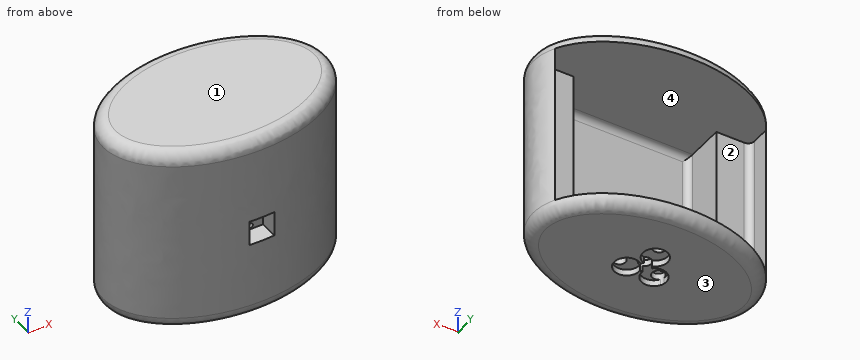
```python
from build123d import *

# Parameters (mm, degrees)
SKETCH1_RX               = 22.86
SKETCH1_RY               = 15.24
BOSS_EXTRUDE4_DEPTH      = 45.72
CUT_EXTRUDE2_START       = -10.16
SKETCH4_W                = 29.21
SKETCH4_H                = 17.78
CUT_EXTRUDE2_DEPTH       = 33.02
SKETCH7_W                = 14.643913221
SKETCH7_H                = 35.56
CUT_EXTRUDE4_DEPTH       = 33.02
CUT_EXTRUDE4_DEPTH_BACK  = 33.02
SKETCH8_R                = 1.27
CUT_EXTRUDE5_DEPTH       = 2.54
FILLET1_R                = 2.54
FILLET2_R                = 2.54
CUT_EXTRUDE11_START      = -2.54
SKETCH12_W               = 43.18
SKETCH12_H               = 19.05
CUT_EXTRUDE11_DEPTH      = 33.02
FILLET3_R                = 1.27
CUT_EXTRUDE13_START      = -2.54
SKETCH13_W               = 5.08
SKETCH13_H               = 5.08
CUT_EXTRUDE13_DEPTH      = 4.8100001
SKETCH14_R               = 0.5
CUT_EXTRUDE14_DEPTH      = 4.8100001
CUT_EXTRUDE14_DEPTH_BACK = 27.6700001
SKETCH16_R               = 2.54
CUT_EXTRUDE15_DEPTH      = 1.27
FILLET4_R                = 1.27


with BuildPart() as part:
    # Sketch1 → Boss-Extrude4 (new body)
    with BuildSketch(Plane.XY):
        with Locations(Location((0, 0), (0, 0, 180))):
            Ellipse(SKETCH1_RX, SKETCH1_RY)
    extrude(amount=BOSS_EXTRUDE4_DEPTH)

    # Sketch4 → Cut-Extrude2 (cut)
    with BuildSketch(Plane.XY.offset(45.72).offset(CUT_EXTRUDE2_START)):
        Rectangle(SKETCH4_W, SKETCH4_H)
    extrude(amount=-CUT_EXTRUDE2_DEPTH, mode=Mode.SUBTRACT)

    # Sketch7 → Cut-Extrude4 (cut, two sides)
    with BuildSketch(Plane(origin=(0, 0, 0), x_dir=(0, 0, -1), z_dir=(1, 0, 0))) as cut_extrude4_sk:
        with Locations((-45.421956611, -1.677648267)):
            Rectangle(SKETCH7_W, SKETCH7_H)
    extrude(amount=CUT_EXTRUDE4_DEPTH, mode=Mode.SUBTRACT)
    extrude(cut_extrude4_sk.sketch, amount=-CUT_EXTRUDE4_DEPTH_BACK, mode=Mode.SUBTRACT)

    # Sketch8 → Cut-Extrude5 (cut)
    with BuildSketch(Plane.XY):
        Circle(SKETCH8_R)
        with Locations((3.998447315, -1.999223657)):
            Circle(SKETCH8_R)
        with Locations((-3.998447315, -1.999223657)):
            Circle(SKETCH8_R)
        with Locations((0, 4.572)):
            Circle(SKETCH8_R)
    extrude(amount=CUT_EXTRUDE5_DEPTH, mode=Mode.SUBTRACT)

    # Fillet1
    fillet1_edges = [part.edges().sort_by_distance(p)[0] for p in [
        (22.859987041, 0.016227247, 0),
    ]]
    fillet(fillet1_edges, radius=FILLET1_R)

    # Fillet2
    fillet2_edges = [part.edges().sort_by_distance(p)[0] for p in [
        (22.860000074, 1.7e-08, 38.1),
    ]]
    fillet(fillet2_edges, radius=FILLET2_R)

    # Sketch12 → Cut-Extrude11 (cut)
    with BuildSketch(Plane(origin=(0, 0, 0), x_dir=(-1, 0, 0), z_dir=(0, 0, -1)).offset(CUT_EXTRUDE11_START)):
        with Locations((0, 9.525)):
            Rectangle(SKETCH12_W, SKETCH12_H)
    extrude(amount=-CUT_EXTRUDE11_DEPTH, mode=Mode.SUBTRACT)

    # Fillet3
    fillet3_edges = [part.edges().sort_by_distance(p)[0] for p in [
        (14.605, -8.89, 19.05),
        (0, -8.89, 35.56),
        (-14.605, -8.89, 19.05),
        (0, -8.89, 2.54),
    ]]
    fillet(fillet3_edges, radius=FILLET3_R)

    # Sketch13 → Cut-Extrude13 (cut, through all)
    with BuildSketch(Plane(origin=(0, -8.89, 0), x_dir=(1, 0, 0), z_dir=(0, 1, 0)).offset(CUT_EXTRUDE13_START)):
        with Locations((0, -18.288)):
            Rectangle(SKETCH13_W, SKETCH13_H)
    extrude(amount=-CUT_EXTRUDE13_DEPTH, mode=Mode.SUBTRACT)

    # Sketch14 → Cut-Extrude14 (cut, two sides)
    with BuildSketch(Plane.XZ.offset(11.43)) as cut_extrude14_sk:
        with Locations((0, 20.077999976)):
            Circle(SKETCH14_R)
        with Locations((0, 16.498)):
            Circle(SKETCH14_R)
    extrude(amount=CUT_EXTRUDE14_DEPTH, mode=Mode.SUBTRACT)
    extrude(cut_extrude14_sk.sketch, amount=-CUT_EXTRUDE14_DEPTH_BACK, mode=Mode.SUBTRACT)

    # Sketch16 → Cut-Extrude15 (cut)
    with BuildSketch(Plane(origin=(0, 0, 0), x_dir=(-1, 0, 0), z_dir=(0, 0, -1))):
        with Locations((2.7942426, -1.505997915)):
            Circle(SKETCH16_R)
        with Locations((0.000242604, 3.333352043)):
            Circle(SKETCH16_R)
        with Locations((-2.793757393, -1.505997915)):
            Circle(SKETCH16_R)
    extrude(amount=-CUT_EXTRUDE15_DEPTH, mode=Mode.SUBTRACT)

    # Fillet4
    fillet4_edges = [part.edges().sort_by_distance(p)[0] for p in [
        (-21.59, 0, 19.05),
        (21.59, 0, 19.05),
    ]]
    fillet(fillet4_edges, radius=FILLET4_R)


solid = part.part
```
Geometry check sheet. Reference: the model listing, model coordinates, mm. Face numbers are marked on the shaded views. Give positions to 0.01 mm unless a question says otherwise; leave off trailing zeros. Write item = value, one per line. Start each with the question number.
1) Gauge pin test, flat ends, axial feed: pin 1 Ø1.5 at (x, z) = (12, 9) entering from +Y; pin 2 Ø1.1 at (y, z) = (-13, 19.5) entering from -X; pin 3 Ø4 at (x, z) = (5.5, 29) entering from -Y. Record the tip position at first contact, or that the pin passes through.
2) Scan lines: L1, parallel to Z at x = -9, y = 0; L2, parallel to X at y = -5, z = 26 (3 decimals); L3, parallel to Z at x = 0, y = -9.75. Record each from-to range of solid material in increasing order.
3) Draft check along Z on the marked faces 1, 2, 3 and 4. Enter one of: released by +Z, released by -Z, zero draft, split by the parting line, or undercut.
Geometry check:
q1.pin_1 = -8.89
q1.pin_2 = -13.18
q1.pin_3 = -15.06
q2.L1 = 0 to 2.54, 35.56 to 38.1
q2.L2 = -21.595 to -14.605, 14.605 to 21.595
q2.L3 = 0 to 16, 17 to 19.58, 20.58 to 38.1
q3.face_1 = released by +Z
q3.face_2 = undercut
q3.face_3 = released by -Z
q3.face_4 = undercut
